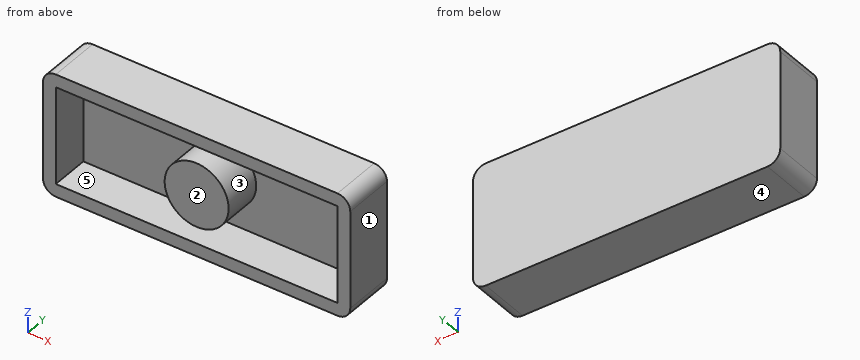
from build123d import *

# Parameters (mm, degrees)
SKETCH1_W           = 15.24
SKETCH1_H           = 6.096
BOSS_EXTRUDE1_DEPTH = 2.54
SHELL1_T            = -0.635
FILLET1_R           = 0.635
SKETCH2_R           = 1.5875
BOSS_EXTRUDE2_DEPTH = 1.905


with BuildPart() as part:
    # Sketch1 → Boss-Extrude1 (new body)
    with BuildSketch(Plane(origin=(0, 0, 0), x_dir=(1, 0, 0), z_dir=(0, 1, 0))):
        with Locations((7.62, 3.048)):
            Rectangle(SKETCH1_W, SKETCH1_H)
    extrude(amount=BOSS_EXTRUDE1_DEPTH)

    # Shell1
    shell1_openings = [part.faces().sort_by_distance(p)[0] for p in [
        (7.62, 0, -3.048),
    ]]
    offset(amount=SHELL1_T, openings=shell1_openings, kind=Kind.INTERSECTION)

    # Fillet1
    fillet1_edges = [part.edges().sort_by_distance(p)[0] for p in [
        (0, 1.27, 0),
        (15.24, 1.27, 0),
        (15.24, 1.27, -6.096),
        (0, 1.27, -6.096),
    ]]
    fillet(fillet1_edges, radius=FILLET1_R)

    # Sketch2 → Boss-Extrude2 (add)
    with BuildSketch(Plane.XZ.offset(-1.905)):
        with Locations(Location((7.62, -3.048, 0), (0, 0, 270))):
            Circle(SKETCH2_R)
    extrude(amount=BOSS_EXTRUDE2_DEPTH)


solid = part.part
CAD build for the part. Positions are in the model's coordinates, mm. Face numbers are marked on the shaded views. A direction names the side the tool comes from. Give positions to 0.01 mm unless a question says otherwise; leave off trailing zeros. Order: outer loops, then holes, each group sorted by start corner. A loop starts at its lowest first (then second) coordinate and runs counter-clockwise, first axis right, second up. Notation, with made-up numbers: (39.5, -26) - (53.5, -26) arc R22 ccw to (53.5, -8) - close; hole circle Ø10 at (70, 77.5). An arc over 180 degrees is marked (long way). Answer in a Markdown table with one row per item.
1. Saw through at A-A, the plane y = 1.45. Give the cut face in (x, z) (1 decimal).
Data:
| item | result |
|---|---|
| outline | (0, -5.5) arc R0.6 ccw to (0.6, -6.1) - (14.6, -6.1) arc R0.6 ccw to (15.2, -5.5) - (15.2, -0.6) arc R0.6 ccw to (14.6, 0) - (0.6, 0) arc R0.6 ccw to (0, -0.6) - close; circle Ø3.2 at (7.6, -3); hole (0.6, -5.5) - (14.6, -5.5) - (14.6, -0.6) - (0.6, -0.6) - close |
2. Saw through at D-D, the plane x = 4.5. Give the cut face in (y, z) (3 decimals), plus the area to 3 significant figures.
Data:
| item | result |
|---|---|
| outline | (0, -6.096) - (2.54, -6.096) - (2.54, 0) - (0, 0) - (0, -0.635) - (1.905, -0.635) - (1.905, -5.461) - (0, -5.461) - close |
| area | 6.29 mm² |
3. Saw through at B-B, the plane z = -1. Give the cut face in (x, y) (3 decimals), plus the area to 3 significant figures.
Data:
| item | result |
|---|---|
| outline | (0, 0) - (0.635, 0) - (0.635, 1.905) - (14.605, 1.905) - (14.605, 0) - (15.24, 0) - (15.24, 2.54) - (0, 2.54) - close |
| area | 12.1 mm² |
4. Pull direction X, two halves, no side cores. Call the marked faces 1, 2 and 3: pulls with the +X half, pulls with the -X half, needs draft (parallel to the pull), parting line crosses it, or undercut.
Data:
| item | result |
|---|---|
| face 1 | pulls with the +X half |
| face 2 | needs draft |
| face 3 | undercut |
5. Tool access for the marked faces 4 and 5: list every direction of +Z, -Z, +X, -X, +Y, -Y with a clear straight run to the whole face (end or side of a thin tool).
Data:
| item | result |
|---|---|
| face 4 | -Z, +X, -X, +Y, -Y |
| face 5 | -Y |
6. Probe probe 1 along X at (y, z) = (0.95, -4.75) (3 decimals); probe 2 along X at (y, z) = (1.35, -4) (3 decimals); probe 3 along X at (y, z) = (0.1, -3.75) (3 decimals). List the from-to ranges inside material, lowest first. Write a range as [from, to].
Data:
| item | result |
|---|---|
| probe 1 | x = [0, 0.635], [14.605, 15.24] |
| probe 2 | x = [0, 0.635], [6.35, 8.89], [14.605, 15.24] |
| probe 3 | x = [0, 0.635], [6.196, 9.044], [14.605, 15.24] |
7. Flat gauge pin, fed straight in: pin 1 (1 mm diameter, centred on x = 2, z = -1.5, fed in from -Y) (3 decimals). Where does the tip first touch, or does it go through?
Data:
| item | result |
|---|---|
| pin 1 | stops at y = 1.905 |
8. Saw through at C-C, the plane x = 7.62. Give the cut face in (y, z) (1 decimal), plus the area to 3 significant figures.
Data:
| item | result |
|---|---|
| outline | (0, -6.1) - (2.5, -6.1) - (2.5, 0) - (0, 0) - (0, -0.6) - (1.9, -0.6) - (1.9, -1.5) - (0, -1.5) - (0, -4.6) - (1.9, -4.6) - (1.9, -5.5) - (0, -5.5) - close |
| area | 12.3 mm² |
